Part model, mm, in its own coordinate system. A direction names the side the tool comes from. Round coordinates to 2 decimals unless told otherwise and drop trailing zeros. Write each loop counter-clockwise with the first axis right and the second up, starting at its lowest first coordinate (ties: lowest second). Pieces come first, ordered by that corner, then holes. Notation, with made-up numbers: (20.5, -29) -> (62.5, -29) arc R21 ccw to (62.5, -15) -> close; hole circle Ø5 at (74, 36.5). An arc over 180 degrees is marked (long way). Return JSON: item names as keys, results as strings. Group by question number.
```python
from build123d import *

# Parameters (mm, degrees)
SKETCH1_W           = 350
SKETCH1_H           = 50
BOSS_EXTRUDE1_DEPTH = 30
CUT_EXTRUDE1_DEPTH  = 10
SKETCH3_R           = 77.5
CUT_EXTRUDE2_DEPTH  = 10
SKETCH4_R           = 12.25
BOSS_EXTRUDE2_DEPTH = 50


with BuildPart() as part:
    # Sketch1 → Boss-Extrude1 (new body)
    with BuildSketch(Plane(origin=(0, 0, 0), x_dir=(0, 0, -1), z_dir=(1, 0, 0))):
        Rectangle(SKETCH1_W, SKETCH1_H)
    extrude(amount=BOSS_EXTRUDE1_DEPTH)

    # Sketch2 → Cut-Extrude1 (cut)
    with BuildSketch(Plane(origin=(30, 0, 0), x_dir=(0, 0, -1), z_dir=(1, 0, 0))):
        with BuildLine():
            Line((155, -6.5), (75, -6.5))
            ThreePointArc((75, -6.5), (68.5, 0), (75, 6.5))
            Line((75, 6.5), (155, 6.5))
            ThreePointArc((155, 6.5), (161.5, 0), (155, -6.5))
        make_face()
    extrude(amount=-CUT_EXTRUDE1_DEPTH, mode=Mode.SUBTRACT)

    # Sketch3 → Cut-Extrude2 (cut)
    with BuildSketch(Plane(origin=(30, 0, 0), x_dir=(0, 0, -1), z_dir=(1, 0, 0))):
        with Locations((-140, 0)):
            Circle(SKETCH3_R)
    extrude(amount=-CUT_EXTRUDE2_DEPTH, mode=Mode.SUBTRACT)

    # Sketch4 → Boss-Extrude2 (add)
    with BuildSketch(Plane(origin=(20, 0, 0), x_dir=(0, 0, -1), z_dir=(1, 0, 0))):
        with Locations((-140, 0)):
            Circle(SKETCH4_R)
    extrude(amount=BOSS_EXTRUDE2_DEPTH)


solid = part.part
```
Item 1: Cut at C-C (y = 0). Write the cut outline in (x, z), then the cut area to 3 significant figures.
Item 2: Cut at D-D (x = 54). Write the cut outline in (y, z).
Item 3: Wall check: L1, parallel to Y at x = 23.5, z = -101; L2, parallel to X at y = 22.5, z = -24; L3, parallel to Z at x = 39, y = -0.5. Give the ranges that are in metal, low to high.
Item 4: Which spindle directions (+Z, -Z, +X, -X, +Y, -Y) get a long thin tool onto all of the face, cutting with end or side? Do faces 4 (the face through (70, 0, 140)), 5 (the face through (30, 0, -52)), 6 (the face through (25.1, 0.1, -161.5)). Say none if no direction does.
Item 5: Two-plate mould, pull along Z, no slides. Class faces 1 (the face through (10, 0, 175)), 2 (the face through (15, 0, -175)), 3 (the face through (20, 0, -116)): released by +Z, released by -Z, zero draft, split by the parting line, or undercut.
Item 6: Flat gauge pins, fed straight in: P1, Ø4, axis at x = 51, y = 5, coming from the -Z side; P2, Ø5, axis at y = 14.5, z = 13.5, coming from the +X side; P3, Ø2, axis at y = 3, z = 78, coming from the +X side. Where does each tip first touch, or does it go through?
Item 7: Cut at B-B (z = 140). Write the cut outline in (x, y).
Item 8: Cut at A-A (x = 25.5). Write the cut outline in (y, z), then the cut area to 3 significant figures.
Checks:
{
 "1": {"outline": "(0, -175) -> (30, -175) -> (30, -161.5) -> (20, -161.5) -> (20, -68.5) -> (30, -68.5) -> (30, 62.5) -> (20, 62.5) -> (20, 127.75) -> (70, 127.75) -> (70, 152.25) -> (20, 152.25) -> (20, 175) -> (0, 175) -> close", "area": "9,670 mm2"},
 "2": {"outline": "circle Ø24.5 at (0, 140)"},
 "3": {"L1": "y = -25 to -6.5, 6.5 to 25", "L2": "x = 0 to 30", "L3": "z = 127.76 to 152.24"},
 "4": {"face 4": "+Z, -Z, +X, +Y, -Y", "face 5": "-Z, +X, +Y, -Y", "face 6": "+X"},
 "5": {"face 1": "released by +Z", "face 2": "released by -Z", "face 3": "undercut"},
 "6": {"P1": "stops at z = 128.12", "P2": "stops at x = 30", "P3": "stops at x = 20"},
 "7": {"outline": "(0, -25) -> (20, -25) -> (20, -12.25) -> (70, -12.25) -> (70, 12.25) -> (20, 12.25) -> (20, 25) -> (0, 25) -> close"},
 "8": {"outline": "(-25, -175) -> (25, -175) -> (25, 66.64) arc R77.5 cw to (-25, 66.64) -> close; circle Ø24.5 at (0, 140); hole (-6.5, -155) arc R6.5 ccw to (6.5, -155) -> (6.5, -75) arc R6.5 ccw to (-6.5, -75) -> close", "area": "11,200 mm2"}
}
